```python
from build123d import *

# Parameters (mm, degrees)
F0_R     = 39.116
F1_DEPTH = 25.4
F2_T     = -2.54
F3_R     = 32.766
F4_DEPTH = 25.4


with BuildPart() as f1:
    # F0 (on Top) → F1 (new body)
    with BuildSketch(Plane.XY):
        Circle(F0_R)
    extrude(amount=F1_DEPTH)

    # F2
    f2_openings = [f1.faces().sort_by_distance(p)[0] for p in [
        (0, 0, 25.4),
    ]]
    offset(amount=F2_T, openings=f2_openings)

    # F3 (on face) → F4 (cut)
    with BuildSketch(Plane(origin=(0, 0, 0), x_dir=(1, 0, 0), z_dir=(0, 0, -1))):
        Circle(F3_R)
    extrude(amount=-F4_DEPTH, mode=Mode.SUBTRACT)


solid = f1.part
```
Read the model definition and answer for the solid it produces. Units are mm, in the model's axes. A direction names the side the tool comes from. Round coordinates to 2 decimals unless told otherwise and drop trailing zeros. Write each loop counter-clockwise with the first axis right and the second up, starting at its lowest first coordinate (ties: lowest second). Pieces come first, ordered by that corner, then holes. Notation, with made-up numbers: (56.25, -4.75) - (93.25, -4.75) arc R18 cw to (93.25, 16.25) - close; hole circle Ø4 at (-26, -17.5). An arc over 180 degrees is marked (long way). One line per item, written item: value.
Q1. For a pull along Y with two mould halves and no side action, classify faces 3 (the flat face through (26, -26, 25.4)), 4 (the cylindrical face through (-7.929, -35.706, 13.81)), 5 (the cylindrical face through (-8.48, -38.186, 12.522)) as pulls with the +Y half, pulls with the -Y half, needs draft (parallel to the pull), parting line crosses it, or undercut.
The answers:
face 3: needs draft
face 4: undercut
face 5: parting line crosses it
Q2. Which of the six approach directions +Z, -Z, +X, -X, +Y, -Y give full straight-line access (tool end or side, diameter ignored) to faces 1 (the flat face through (-9, -32, 0)), 2 (the flat face through (-33, -3, 2.54))?
The answers:
face 1: -Z, +X, -X, +Y, -Y
face 2: +Z
Q3. Each of these flat-tipped pins is pushed along its axis until it touches: P1, Ø10, axis at x = -21, z = 15.5, coming from the -Y side; P2, Ø1, axis at y = -12.5, z = 19.5, coming from the +X side; P3, Ø4, axis at y = -30, z = 7.5, coming from the -X side. Where does it stop, or does it pass through?
The answers:
P1: stops at y = -35.69
P2: stops at x = 37.23
P3: stops at x = -27.31
Q4. Find section C-C (z = 14.75). Determine the outline of the cut face in (x, y).
The answers:
outline: circle Ø78.23 at (0, 0); hole circle Ø73.15 at (0, 0)
Q5. Find section A-A (x = 0). Determine the outline of the cut face in (y, z).
The answers:
outline: (-39.12, 0) - (-32.77, 0) - (-32.77, 2.54) - (-36.58, 2.54) - (-36.58, 25.4) - (-39.12, 25.4) - close; (32.77, 0) - (39.12, 0) - (39.12, 25.4) - (36.58, 25.4) - (36.58, 2.54) - (32.77, 2.54) - close
Q6. Straight lines are drawn through the part: line 1 (Y direction, x = 0, z = 1.8); line 2 (Y direction, x = 0, z = 14.75); line 3 (Z direction, x = -3, y = 33). For each, find the intervals that lie inside material, in ascending order. Write a range as from..to.
The answers:
line 1: y = -39.12..-32.77, 32.77..39.12
line 2: y = -39.12..-36.58, 36.58..39.12
line 3: z = 0..2.54
